For this review, take the finished solid that the model builds, in its own axes (mm). Face numbers are marked on the shaded views. A direction names the side the tool comes from. Give positions to 0.01 mm unless a question says otherwise; leave off trailing zeros. Write each loop counter-clockwise with the first axis right and the second up, starting at its lowest first coordinate (ties: lowest second). Pieces come first, ordered by that corner, then holes. Notation, with made-up numbers: M 56,88.5 L 93,88.5 A19 ccw 93,118.5 Z; hole C 11,5.5 d8. An arc over 180 degrees is marked long. Use one line per item in the form item = value. Start each with the question number.
Q1. Consider section B-B on x = 37. Write out the cut boundary in (y, z), and give its area (3 significant figures).
Q2. Clearance check with flat-ended pins moving along their axes: pin 1 Ø10 at (y, z) = (12, 122.5) entering from -X; pin 2 Ø1.5 at (x, z) = (33, 125.5) entering from +Y; pin 3 Ø4 at (x, y) = (22.5, 29) entering from +Z; pin 4 Ø24.5 at (x, z) = (16.5, 123.5) entering from -Y. State where each tip first meets the part, or that it passes through.
Q3. For probe 1 along Z at (x, y) = (5, -17.5); probe 2 along Y at (x, z) = (5, 92); probe 3 along X at (y, z) = (2.5, 59.5), list the stretches that pass through material, from the lowest coordinate up. Write a range as [from, to].
Q4. Consider section D-D on x = 5. Write out the cut boundary in (y, z).
Q5. Mouldability with a two-part tool opening along X and no side actions: class the marked faces 3, 4 and 5 as released by +X, released by -X, zero draft, split by the parting line, or undercut.
Q6. Consider section A-A on z = 96. Write out the cut boundary in (x, y), and give its area (3 significant figures).
Q7. Tool access review of the marked faces 1 and 2: name each direction out of +Z, -Z, +X, -X, +Y, -Y from which nothing blocks a thin tool from reaching the whole face with its end or side.
Q8. Consider section C-C on y = 38.5. Write out the cut boundary in (x, z).
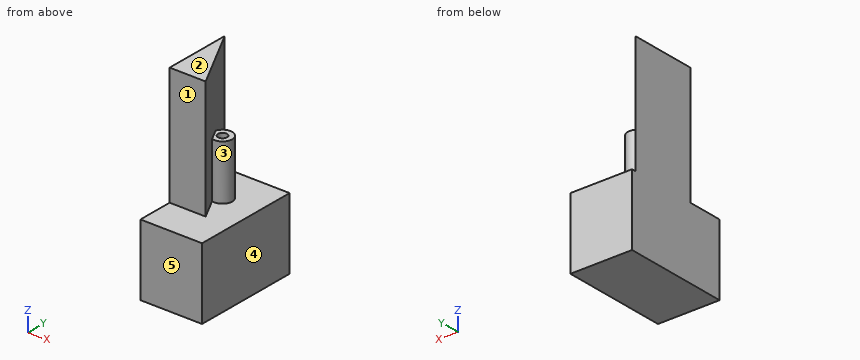
```python
from build123d import *

# Parameters (mm, degrees)
F0_W     = 91.597288847
F0_H     = 60.767069459
F1_DEPTH = 52.9421810061
F2_R     = 8.3288668083
F2_R_2   = 3.9203402896
F3_DEPTH = 46.854743734
F6_DEPTH = 101.6741897911


with BuildPart() as f1:
    # F0 (on Right) → F1 (new body)
    with BuildSketch(Plane.YZ):
        with Locations((15.2086205781, 24.4252681732)):
            Rectangle(F0_W, F0_H)
    extrude(amount=F1_DEPTH)

    # F2 (on face) → F3 (join)
    with BuildSketch(Plane.XY.offset(54.8088029027)):
        with Locations((22.8059887886, 27.5532379746)):
            Circle(F2_R)
        with Locations((22.8059887886, 27.5532379746)):
            Circle(F2_R_2, mode=Mode.SUBTRACT)
    extrude(amount=F3_DEPTH)

    # F5 (on face) → F6 (join)
    with BuildSketch(Plane.XY.offset(54.8088029027)):
        Polygon((0, 0), (30.9126600623, 0), (0, 57.6490387321), align=None)
    extrude(amount=F6_DEPTH)


solid = f1.part
```
Working result:
q1.outline = M -30.59,-5.96 L 61.01,-5.96 L 61.01,54.81 L -30.59,54.81 Z
q1.area = 5,570 mm²
q2.pin_1 = 0
q2.pin_2 = through
q2.pin_3 = 54.81
q2.pin_4 = 0
q3.probe_1 = [-5.96, 54.81]
q3.probe_2 = [0, 48.32]
q3.probe_3 = [0, 29.57]
q4.outline = M -30.59,-5.96 L 61.01,-5.96 L 61.01,54.81 L 48.32,54.81 L 48.32,156.48 L 0,156.48 L 0,54.81 L -30.59,54.81 Z
q5.face_3 = undercut
q5.face_4 = released by +X
q5.face_5 = zero draft
q6.outline = M 0,0 L 30.91,0 L 20.42,19.57 A8.33 ccw long 14.84,29.98 L 0,57.65 Z; hole C 22.81,27.55 d7.84
q6.area = 1,040 mm²
q7.face_1 = +Z, +X, -X, -Y
q7.face_2 = +Z, +X, -X, +Y, -Y
q8.outline = M 0,-5.96 L 52.94,-5.96 L 52.94,54.81 L 10.27,54.81 L 10.27,156.48 L 0,156.48 Z
